from build123d import *

# Parameters (mm, degrees)
F0_R     = 7.5
F1_DEPTH = 15
F2_R     = 8.8984666771
F2_R_2   = 7.5
F3_DEPTH = 2
F4_T     = 2.5


# Not quite as in the source:
# - a fillet or chamfer that OpenCascade refuses, or shapes differently, is made with other operations: its cross-section is extruded or revolved along the edge and cut away or added
# - a shell that OpenCascade refuses in one call is made with other operations: the cavity is built on its own and cut out


with BuildPart() as f1:
    # F0 (on Top) → F1 (new body)
    with BuildSketch(Plane.XY):
        Circle(F0_R)
    extrude(amount=F1_DEPTH)

    # F2 (on face) → F3 (join)
    with BuildSketch(Plane.XY):
        Circle(F2_R)
        Circle(F2_R_2, mode=Mode.SUBTRACT)
    extrude(amount=F3_DEPTH)

    # F4: shell of thickness 2.5, made by hand


with BuildPart() as f4_core1:
    # F4_t2: copy of F1
    add(f1.part)

    # the walls: a layer under each face that stays
    f4_faces = [f4_core1.faces().sort_by_distance(p)[0] for p in [
        (-7.5, 0, 8.5),
        (-5.9323111181, -5.9323111181, 2),
        (-8.8984666771, 0, 1),
    ]]
    thicken(f4_faces, amount=-F4_T, mode=Mode.SUBTRACT)

    # F4_s3 → F4_t4 (revolve, cut)
    with BuildSketch(Plane.XZ):
        Polygon((7.525, 2.025), (5, 2), (5, -0.5), (7.5, -0.5), align=None)
    revolve(axis=Axis((0, 0, 2), (0, 0, 1)), mode=Mode.SUBTRACT)


with BuildPart() as f1_1:
    add(f1.part)

    # what is left inside the walls is the cavity
    f4_cavity = [f4_core1.part.solids().sort_by_distance(p)[0] for p in [
        (-4.975, 0, 10),
    ]]
    add(f4_cavity, mode=Mode.SUBTRACT)

    # F5: fillet of radius 3 on 1 edges, made by hand

    # F5_s1 → F5_t2 (revolve, cut)
    with BuildSketch(Plane.XZ):
        with BuildLine():
            ThreePointArc((7.5, 12.0419601084), (6.7912878475, 13.9784517816), (5, 15))
            Line((5, 15), (7.5, 15))
            Line((7.5, 15), (7.5, 12.0419601084))
        make_face()
    revolve(axis=Axis((0, 0, 15), (0, 0, 1)), mode=Mode.SUBTRACT)


solid = f1_1.part
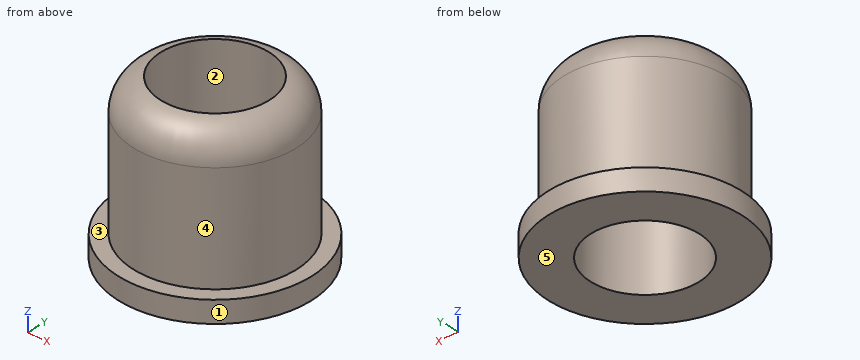
The listing builds one solid part. Answer for the finished solid, in the listing's coordinates (mm). Face numbers are marked on the shaded views. A direction names the side the tool comes from. Give positions to 0.01 mm unless a question says otherwise; leave off trailing zeros. Order: outer loops, then holes, each group sorted by start corner. A loop starts at its lowest first (then second) coordinate and runs counter-clockwise, first axis right, second up. Notation, with made-up numbers: (47, -25) - (79, -25) arc R10 cw to (79, -14) - close; hole circle Ø11 at (31.25, 6.5). An arc over 180 degrees is marked (long way). One line per item, written item: value. Start each with the question number.
1) The mould has two halves that part along X. Classify the marked faces 1, 2 and 3: released by +X, released by -X, zero draft, split by the parting line, or undercut.
2) A tool of negligible diameter and unlimited length cuts with its end or side. For the marked faces 4 and 5, from which of +Z, -Z, +X, -X, +Y, -Y can it reach the whole face along a straight path? Write none if from no direction.
3) A cutting plane is placed at A-A on x = 0. Give the vertices of the cut face in (y, z).
4) Given pin 1 Ø8 at (y, z) = (-7, 10) entering from -X; pin 2 Ø5 at (x, z) = (0, 11.5) entering from -Y; pin 3 Ø1 at (x, z) = (-6.5, 11.5) entering from +Y; pin 4 Ø4 at (x, y) = (1, -1.5) entering from -Z, each flat-ended and moving along its own axis, determine where each tip first touches the part or whether it passes through.
5) A cutting plane is placed at C-C on z = 9.5. Give the vertices of the cut face in (x, y).
6) Find the intervals of material crossed by L1, parallel to Y at x = 0, z = 8.5; L2, parallel to X at y = -0.5, z = 10.75; L3, parallel to X at y = 3.25, z = 4.75, in increasing order.
Answer sheet:
1. face 1: split by the parting line
1. face 2: undercut
1. face 3: zero draft
2. face 4: +Z
2. face 5: -Z, +X, -X, +Y, -Y
3. outline: (-8.9, 0) - (-5, 0) - (-5, 15) arc R3 ccw to (-7.5, 12.04) - (-7.5, 2) - (-8.9, 2) - close; (5, 0) - (8.9, 0) - (8.9, 2) - (7.5, 2) - (7.5, 12.04) arc R3 ccw to (5, 15) - close
4. pin 1: stops at x = -6.87
4. pin 2: stops at y = -7.5
4. pin 3: stops at y = 4.5
4. pin 4: passes through
5. outline: circle Ø15 at (0, 0); hole circle Ø10 at (0, 0)
6. L1: y = -7.5 to -5, 5 to 7.5
6. L2: x = -7.48 to -4.97, 4.97 to 7.48
6. L3: x = -6.76 to -3.8, 3.8 to 6.76
